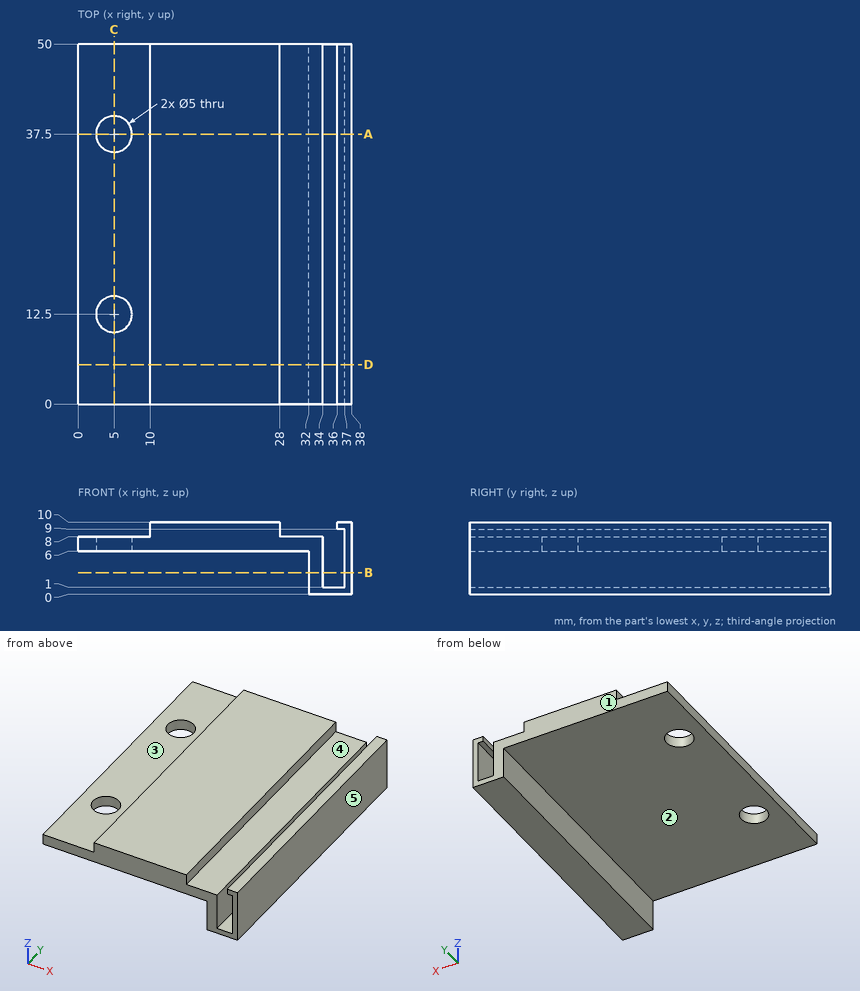
Geometry check sheet. Reference: drawing and pictorial views, mm from the part's lowest x, y, z. A direction names the side the tool comes from. Coordinates: 2 decimals unless noted, no trailing zeros. Order: outer loops, then holes, each group sorted by start corner. A loop starts at its lowest first (then second) coordinate and runs counter-clockwise, first axis right, second up.
Item 1: Material ranges on L1, parallel to Y at x = 5, z = 7.3; L2, parallel to Z at x = 36.5, y = 26.5; L3, parallel to X at y = 11, z = 5.5, recorded low to high.
Filled in:
L1: y = 0 to 10, 15 to 35, 40 to 50
L2: z = 0 to 1, 9 to 10
L3: x = 32 to 34, 37 to 38
Item 2: Section check A-A, the plane y = 37.5. Enter the section's corners in (x, z).
Filled in:
outline: (0, 6) - (2.5, 6) - (2.5, 8) - (0, 8) - close; (7.5, 6) - (32, 6) - (32, 0) - (38, 0) - (38, 10) - (36, 10) - (36, 9) - (37, 9) - (37, 1) - (34, 1) - (34, 8) - (28, 8) - (28, 10) - (10, 10) - (10, 8) - (7.5, 8) - close
Item 3: Section check D-D, the plane y = 5.5. Enter the section's corners in (x, z), then the cut area to 3 significant figures.
Filled in:
outline: (0, 6) - (32, 6) - (32, 0) - (38, 0) - (38, 10) - (36, 10) - (36, 9) - (37, 9) - (37, 1) - (34, 1) - (34, 8) - (28, 8) - (28, 10) - (10, 10) - (10, 8) - (0, 8) - close
area: 130 mm2
Item 4: Depth check by flat-ended pin: pin 1 (1 mm diameter, centred on x = 16.5, z = 4, fed in from -Y); pin 2 (3 mm diameter, centred on x = 6.5, y = 33, fed in from +Z); pin 3 (12 mm diameter, centred on x = 12, y = 44.5, fed in from -Z); pin 4 (0.5 mm diameter, centred on y = 35, z = 9.5, fed in from -X). Enter the tip coordinate at first touch or a pass-through.
Filled in:
pin 1: passes through
pin 2: stops at z = 8
pin 3: stops at z = 6
pin 4: stops at x = 10
Item 5: Section check B-B, the plane z = 3. Enter the section's corners in (x, y), then the cut area to 3 significant figures.
Filled in:
outline: (32, 0) - (34, 0) - (34, 50) - (32, 50) - close; (37, 0) - (38, 0) - (38, 50) - (37, 50) - close
area: 150 mm2
Item 6: Release check for a two-part mould opening along X. For the marked faces 3, 4 and 5 record: +X half, -X half, draft (parallel to the pull), parting line (faces both ways), or undercut.
Filled in:
face 3: draft
face 4: undercut
face 5: +X half
Item 7: Section check C-C, the plane x = 5. Enter the section's corners in (y, z), then the cut area to 3 significant figures.
Filled in:
outline: (0, 6) - (10, 6) - (10, 8) - (0, 8) - close; (15, 6) - (35, 6) - (35, 8) - (15, 8) - close; (40, 6) - (50, 6) - (50, 8) - (40, 8) - close
area: 80.0 mm2
Item 8: Access from +Z, -Z, +X, -X, +Y, -Y to the whole of each face (thin tool, end or side, straight path). Record for the marked faces 1 and 2.
Filled in:
face 1: +Z, -Z, +X, -X, +Y
face 2: -Z, -X, +Y, -Y
